Read the model definition and answer for the solid it produces. Units are mm, in the model's axes. Coordinates: 2 decimals unless noted, no trailing zeros. Loops run counter-clockwise (first coordinate to the right, second up) from the corner with the lowest first, then second, coordinate; pieces in that order, holes last. Notation, with made-up numbers: M 16,-35 L 44,-35 A18 cw 44,-23 Z; hole C 72,-22 d2. An arc over 180 degrees is marked long. One line per item, written item: value. Start each with the question number.
Autodesk Inventor part; units mm, degrees
ref_plane "YZ Plane" through (0, 0, 0) normal (1, 0, 0) x (0, 1, 0)
ref_plane "XZ Plane" through (0, 0, 0) normal (0, 1, 0) x (-1, 0, 0)
ref_plane "XY Plane" through (0, 0, 0) normal (0, 0, 1) x (1, 0, 0)
sketch "草图1" plane through (0, 0, 0) normal (0, 1, 0) x (-1, 0, 0)
  line L0 (35.3553, 35.3553) -> (-35.3553, 35.3553)
  line L1 (-35.3553, 35.3553) -> (-35.3553, -35.3553)
  line L2 (-35.3553, -35.3553) -> (35.3553, -35.3553)
  line L3 (35.3553, -35.3553) -> (35.3553, 35.3553)
  line L4 (35.3553, 35.3553) -> (-35.3553, -35.3553)
  line L5 (35.3553, -35.3553) -> (-35.3553, 35.3553)
  line L6 (-24.7487, 45.9619) -> (-45.9619, 24.7487)
  line L7 (-45.9619, -24.7487) -> (-24.7487, -45.9619)
  line L8 (24.7487, -45.9619) -> (45.9619, -24.7487)
  line L9 (45.9619, 24.7487) -> (24.7487, 45.9619)
  line L10 (24.7487, 45.9619) -> (-24.7487, 45.9619)
  line L11 (45.9619, 24.7487) -> (45.9619, -24.7487)
  line L12 (24.7487, -45.9619) -> (-24.7487, -45.9619)
  line L13 (-45.9619, -24.7487) -> (-45.9619, 24.7487)
  circle A0 centre (41.0122, 25.4558) radius 1.65
  circle A1 centre (27.5772, 27.5772) radius 1.65
  circle A2 centre (25.4558, 41.0122) radius 1.65
  circle A3 centre (-25.4558, 41.0122) radius 1.65
  circle A4 centre (-27.5772, 27.5772) radius 1.65
  circle A5 centre (-41.0122, 25.4558) radius 1.65
  circle A6 centre (-41.0122, -25.4558) radius 1.65
  circle A7 centre (-27.5772, -27.5772) radius 1.65
  circle A8 centre (-25.4558, -41.0122) radius 1.65
  circle A9 centre (25.4558, -41.0122) radius 1.65
  circle A10 centre (27.5772, -27.5772) radius 1.65
  circle A11 centre (41.0122, -25.4558) radius 1.65
  point P0 (0, 0)
  point P1 (0, 0)
  point P2 (-35.3553, -35.3553)
  point P3 (35.3553, -35.3553)
  dimension "d0" = 100
  dimension "d1" = 30
  dimension "d2" = 45
  dimension "d5" = 360
  dimension "d12" = 3.3
  dimension "d13" = 3
  dimension "d14" = 11
  dimension "d15" = 3.3
  dimension "d16" = 11
  dimension "d19" = 360
extrude "拉伸1" add sketch "草图1" along normal blind 3 contours L4 A1 L5 A4 L0 | L9 L11 L8 L3 | L3 L5 A10 L4 A1 | L0 L6 L10 L9 | L5 A4 L4 A7 L1 | L1 L7 L13 L6 | L8 L12 L7 L2 | L2 L4 A7 L5 A10
sketch "草图2" plane through (0, 3, 0) normal (0, 1, 0) x (1, 0, 0)
  line L0 (45.9619, -24.7487) -> (45.9619, 24.7487)
  line L1 (45.9619, 24.7487) -> (24.7487, 45.9619)
  line L2 (24.7487, 45.9619) -> (-24.7487, 45.9619)
  line L3 (-24.7487, 45.9619) -> (-45.9619, 24.7487)
  line L4 (-45.9619, 24.7487) -> (-45.9619, -24.7487)
  line L5 (-45.9619, -24.7487) -> (-24.7487, -45.9619)
  line L6 (-24.7487, -45.9619) -> (24.7487, -45.9619)
  line L7 (24.7487, -45.9619) -> (45.9619, -24.7487)
  circle A0 centre (27.5772, 27.5772) radius 1.65
  circle A1 centre (-27.5772, 27.5772) radius 1.65
  circle A2 centre (25.4558, -41.0122) radius 1.65
  circle A3 centre (-25.4558, -41.0122) radius 1.65
  circle A4 centre (-41.0122, 25.4558) radius 1.65
  circle A5 centre (-41.0122, -25.4558) radius 1.65
  circle A6 centre (25.4558, 41.0122) radius 1.65
  circle A7 centre (-25.4558, 41.0122) radius 1.65
  circle A8 centre (-27.5772, -27.5772) radius 1.65
  circle A9 centre (41.0122, -25.4558) radius 1.65
  circle A10 centre (41.0122, 25.4558) radius 1.65
  circle A11 centre (27.5772, -27.5772) radius 1.65
  line L8 (-45.9619, 0) -> (0, 0)
  line L9 (0, 0) -> (45.9619, 0)
  line L10 (0, 0) -> (0, 45.9619)
  line L11 (0, 0) -> (0, -45.9619)
  line L12 (-39.9619, -15) -> (-29.9619, -15)
  line L13 (-29.9619, -15) -> (-29.9619, 15)
  line L14 (-29.9619, 15) -> (-39.9619, 15)
  line L15 (-39.9619, 15) -> (-39.9619, -15)
  line L16 (-20, -16) -> (20, -16)
  line L17 (20, -16) -> (20, -8)
  line L18 (20, -8) -> (-20, -8)
  line L19 (-20, -8) -> (-20, -16)
  line L20 (39.9619, -15) -> (29.9619, -15)
  line L21 (29.9619, -15) -> (29.9619, 15)
  line L22 (29.9619, 15) -> (39.9619, 15)
  line L23 (39.9619, 15) -> (39.9619, -15)
  line L24 (-20, -35.9619) -> (20, -35.9619)
  line L25 (20, -35.9619) -> (20, -27.9619)
  line L26 (20, -27.9619) -> (-20, -27.9619)
  line L27 (-20, -27.9619) -> (-20, -35.9619)
  line L28 (-20, 16) -> (20, 16)
  line L29 (20, 16) -> (20, 8)
  line L30 (20, 8) -> (-20, 8)
  line L31 (-20, 8) -> (-20, 16)
  line L32 (-20, 35.9619) -> (20, 35.9619)
  line L33 (20, 35.9619) -> (20, 27.9619)
  line L34 (20, 27.9619) -> (-20, 27.9619)
  line L35 (-20, 27.9619) -> (-20, 35.9619)
  dimension "d21" = 30
  dimension "d22" = 10
  dimension "d23" = 6
  dimension "d24" = 15
  dimension "d25" = 8
  dimension "d27" = 8
  dimension "d29" = 40
  dimension "d30" = 20
  dimension "d31" = 8
  dimension "d32" = 40
  dimension "d33" = 20
  dimension "d34" = 10
extrude "拉伸2" cut sketch "草图2" against normal through all contours L23 L20 L21 L9 | L9 L21 L22 L23 | L24 L27 L26 L11 | L11 L26 L25 L24 | L32 L33 L34 L10 | L10 L34 L35 L32 | L13 L12 L15 L8 | L8 L15 L14 L13 | L30 L31 L28 L10 | L10 L28 L29 L30 | L18 L17 L16 L11 | L11 L16 L19 L18
fillet "圆角1" radius 5 8 edges at (-39.9619, 1.5, 15) (-29.9619, 1.5, 15) (-39.9619, 1.5, -15) (-29.9619, 1.5, -15) (29.9619, 1.5, -15) (39.9619, 1.5, -15) (39.9619, 1.5, 15) (29.9619, 1.5, 15)
fillet "圆角2" radius 3 16 edges at (-20, 1.5, 35.9619) (-20, 1.5, 27.9619) (20, 1.5, 35.9619) (20, 1.5, 27.9619) (-20, 1.5, 16) (-20, 1.5, 8) (20, 1.5, 16) (20, 1.5, 8) (-20, 1.5, -8) (20, 1.5, -8) (-20, 1.5, -16) (20, 1.5, -16) (-20, 1.5, -27.9619) (-20, 1.5, -35.9619) (20, 1.5, -27.9619) (20, 1.5, -35.9619)
properties part number "上板"
1) Flat-ended cylindrical pins translate along their axes: pin 1 (3 mm diameter, centred on x = 25.46, z = -41.01, fed in from +Y); pin 2 (5.5 mm diameter, centred on x = -27.58, z = 27.58, fed in from +Y); pin 3 (1.6 mm diameter, centred on y = 2, z = -31.5, fed in from -X). Find the tip coordinate at first contact, or state that the pin passes through.
2) Section A-A (z = -1.5) is taken. Determine the outline of the cut face in (x, y), then the cut area to 3 significant figures.
3) Section B-B (x = -6) is taken. Determine the outline of the cut face in (y, z).
4) Consider line 1 along Z through (x, y) = (-16, 2.4); line 2 along Z through (x, y) = (-27.5, 0.15); line 3 along X through (y, z) = (2.9, -41.5). Determine where each line is inside the solid, lowest interval first.
5) For a pull along Z with two mould halves and no side action, classify faces 1 (the face through (19.14, 1.48, -8.9)), 2 (the face through (45.962, 1, 0)) as released by +Z, released by -Z, zero draft, split by the parting line, or undercut.
6) Section C-C (y = 1.3) is taken. Count the separate pieces of the cut face and the enclosed holes in it, then the cut area to 3 significant figures.
Results found:
1. pin 1: passes through
1. pin 2: stops at y = 3
1. pin 3: stops at x = -40.01
2. outline: M -45.96,0 L -39.96,0 L -39.96,3 L -45.96,3 Z; M -29.96,0 L 29.96,0 L 29.96,3 L -29.96,3 Z; M 39.96,0 L 45.96,0 L 45.96,3 L 39.96,3 Z
2. area: 216 mm²
3. outline: M 0,-45.96 L 3,-45.96 L 3,-35.96 L 0,-35.96 Z; M 0,-27.96 L 3,-27.96 L 3,-16 L 0,-16 Z; M 0,-8 L 3,-8 L 3,8 L 0,8 Z; M 0,16 L 3,16 L 3,27.96 L 0,27.96 Z; M 0,35.96 L 3,35.96 L 3,45.96 L 0,45.96 Z
4. line 1: z = -45.96 to -35.96, -27.96 to -16, -8 to 8, 16 to 27.96, 35.96 to 45.96
4. line 2: z = -43.21 to -29.23, -25.93 to 25.93, 29.23 to 43.21
4. line 3: x = -29.21 to -27.03, -23.88 to 23.88, 27.03 to 29.21
5. face 1: undercut
5. face 2: zero draft
6. separate pieces: 1
6. enclosed holes: 18
6. area: 5,640 mm²
